```python
from build123d import *

# Parameters (mm, degrees)
TRIAL_LOAD_PLATE_PROFILE_R           = 13
TRIAL_LOAD_PLATE_PROFILE_R_2         = 4
TRIAL_LOAD_PLATE_DEPTH               = 4
CAPTURED_HORN_KEY_BOSS_START         = -1.65
CAPTURED_HORN_KEY_BOSS_PROFILE_R     = 13
CAPTURED_HORN_KEY_BOSS_DEPTH         = 1.65
KEY_POCKET_HUB_START                 = -1.65
STOCK_HORN_POCKET_HUB_R              = 3.5
KEY_POCKET_HUB_DEPTH                 = 1.65
KEY_POCKET_HORIZONTAL_START          = -1.65
STOCK_HORN_POCKET_HORIZONTAL_W       = 16.3
STOCK_HORN_POCKET_HORIZONTAL_H       = 4.1
KEY_POCKET_HORIZONTAL_DEPTH          = 1.65
KEY_POCKET_VERTICAL_START            = -1.65
STOCK_HORN_POCKET_VERTICAL_W         = 4.1
STOCK_HORN_POCKET_VERTICAL_H         = 16.3
KEY_POCKET_VERTICAL_DEPTH            = 1.65
KEY_POCKET_ROUNDED_TIPS_START        = -1.65
STOCK_HORN_POCKET_ROUNDED_TIPS_R     = 2.05
KEY_POCKET_ROUNDED_TIPS_DEPTH        = 1.65
UNMODIFIED_HORN_CAPTURE_M2_START     = -50
UNMODIFIED_HORN_CAPTURE_M2_PROFILE_R = 1.15
UNMODIFIED_HORN_CAPTURE_M2_DEPTH     = 69.814887722
HUB_CLEARANCE_IN_KEY_BOSS_ONLY_START = -1.65
HORN_CENTER_HUB_CLEARANCE_R          = 4
HUB_CLEARANCE_IN_KEY_BOSS_ONLY_DEPTH = 1.65


with BuildPart() as part:
    # Trial_load_plate_profile → Trial_load_plate (new body)
    with BuildSketch(Plane.XY):
        Circle(TRIAL_LOAD_PLATE_PROFILE_R)
        Circle(TRIAL_LOAD_PLATE_PROFILE_R_2, mode=Mode.SUBTRACT)
    extrude(amount=TRIAL_LOAD_PLATE_DEPTH)

    # Captured_horn_key_boss_profile → Captured_horn_key_boss (add)
    with BuildSketch(Plane.XY.offset(CAPTURED_HORN_KEY_BOSS_START)):
        Circle(CAPTURED_HORN_KEY_BOSS_PROFILE_R)
    extrude(amount=CAPTURED_HORN_KEY_BOSS_DEPTH)

    # Stock_horn_pocket_Hub → Key_pocket_Hub (cut)
    with BuildSketch(Plane.XY.offset(KEY_POCKET_HUB_START)):
        Circle(STOCK_HORN_POCKET_HUB_R)
    extrude(amount=KEY_POCKET_HUB_DEPTH, mode=Mode.SUBTRACT)

    # Stock_horn_pocket_Horizontal → Key_pocket_Horizontal (cut)
    with BuildSketch(Plane.XY.offset(KEY_POCKET_HORIZONTAL_START)):
        Rectangle(STOCK_HORN_POCKET_HORIZONTAL_W, STOCK_HORN_POCKET_HORIZONTAL_H)
    extrude(amount=KEY_POCKET_HORIZONTAL_DEPTH, mode=Mode.SUBTRACT)

    # Stock_horn_pocket_Vertical → Key_pocket_Vertical (cut)
    with BuildSketch(Plane.XY.offset(KEY_POCKET_VERTICAL_START)):
        Rectangle(STOCK_HORN_POCKET_VERTICAL_W, STOCK_HORN_POCKET_VERTICAL_H)
    extrude(amount=KEY_POCKET_VERTICAL_DEPTH, mode=Mode.SUBTRACT)

    # Stock_horn_pocket_Rounded_tips → Key_pocket_Rounded_tips (cut)
    with BuildSketch(Plane.XY.offset(KEY_POCKET_ROUNDED_TIPS_START)):
        with Locations((8.15, 0)):
            Circle(STOCK_HORN_POCKET_ROUNDED_TIPS_R)
        with Locations((-8.15, 0)):
            Circle(STOCK_HORN_POCKET_ROUNDED_TIPS_R)
        with Locations((0, 8.15)):
            Circle(STOCK_HORN_POCKET_ROUNDED_TIPS_R)
        with Locations((0, -8.15)):
            Circle(STOCK_HORN_POCKET_ROUNDED_TIPS_R)
    extrude(amount=KEY_POCKET_ROUNDED_TIPS_DEPTH, mode=Mode.SUBTRACT)

    # Unmodified_horn_capture_M2_profile → Unmodified_horn_capture_M2 (cut, through all)
    with BuildSketch(Plane.XY.offset(UNMODIFIED_HORN_CAPTURE_M2_START)):
        with Locations((7, 7)):
            Circle(UNMODIFIED_HORN_CAPTURE_M2_PROFILE_R)
        with Locations((-7, 7)):
            Circle(UNMODIFIED_HORN_CAPTURE_M2_PROFILE_R)
        with Locations((-7, -7)):
            Circle(UNMODIFIED_HORN_CAPTURE_M2_PROFILE_R)
        with Locations((7, -7)):
            Circle(UNMODIFIED_HORN_CAPTURE_M2_PROFILE_R)
    extrude(amount=UNMODIFIED_HORN_CAPTURE_M2_DEPTH, mode=Mode.SUBTRACT)

    # Horn_center_hub_clearance → Hub_clearance_in_key_boss_only (cut)
    with BuildSketch(Plane.XY.offset(HUB_CLEARANCE_IN_KEY_BOSS_ONLY_START)):
        with Locations(Location((0, 0, 0), (0, 0, 149.169502568))):
            Circle(HORN_CENTER_HUB_CLEARANCE_R)
    extrude(amount=HUB_CLEARANCE_IN_KEY_BOSS_ONLY_DEPTH, mode=Mode.SUBTRACT)


solid = part.part
```
Can you work these out from the model? Positions are in its coordinate system, mm. A direction names the side the tool comes from. Give positions to 0.01 mm unless a question says otherwise; leave off trailing zeros. Order: outer loops, then holes, each group sorted by start corner. A loop starts at its lowest first (then second) coordinate and runs counter-clockwise, first axis right, second up. Notation, with made-up numbers: (76, 46.5) - (116, 46.5) arc R28 cw to (116, 80.5) - close; hole circle Ø9 at (32, 83.5). An arc over 180 degrees is marked (long way). Use a Markdown table: item, result. Add a question column.
Q1. Please list where these lines run through material, in increasing order: line 1 along Y through (x, z) = (-7, 2.1); line 2 along X through (y, z) = (-3, 0.9).
Q2. I'm going to push flat-ended pins straight in: pin 1 (1.8 mm diameter, centred on x = -7, y = 7, fed in from -Z); pin 2 (0.5 mm diameter, centred on y = 6.5, z = -1, fed in from -X); pin 3 (2 mm diameter, centred on x = 1, y = -7, fed in from -Z); pin 4 (1.3 mm diameter, centred on x = -5, z = -0.5, fed in from -Y). Where does each tip first touch, or does it pass through?
Q3. If we section it at B-B on y = 2.75: Write out the boundary of the cut face in (x, z).
Q4. If we mould it in two halves opening along X, with no side actions, what happens to faces 1 (the cylindrical face through (10.2, 0, -0.8)), 2 (the flat face through (3, 3, 4)), 3 (the cylindrical face through (-10.316, -7.91, 1.135))? For each: released by +X, released by -X, zero draft, split by the parting line, or undercut.
Q5. If we section it at D-D on x = -7.5: Write out the boundary of the cut face in (y, z), plus the area to 3 significant figures.
Q6. If we section it at C-C on z = 2.2: Write out the boundary of the cut face in (x, y).
Q7. On a 3-axis mill with a long thin cutter (end or side, diameter ignored), from which of +Z, -Z, +X, -X, +Y, -Y can I reach the whole of each face in a straight line? I mean faces 4 (the cylindrical face through (6.85, -5.86, 1.14)), 5 (the flat face through (-2.05, -6, -1)). Say none if no direction works.
Q8. If we section it at A-A on x = 0: Write out the boundary of the cut face in (y, z).
Answers follow:
| question | item | result |
|---|---|---|
| 1 | line 1 | y = -10.95 to -8.15, -5.85 to 5.85, 8.15 to 10.95 |
| 1 | line 2 | x = -12.65 to -2.65, 2.65 to 12.65 |
| 2 | pin 1 | passes through |
| 2 | pin 2 | stops at x = -11.4 |
| 2 | pin 3 | stops at z = 0 |
| 2 | pin 4 | stops at y = -12.25 |
| 3 | outline | (-12.71, -1.65) - (-2.9, -1.65) - (-2.9, 4) - (-12.71, 4) - close; (2.9, -1.65) - (12.71, -1.65) - (12.71, 4) - (2.9, 4) - close |
| 4 | face 1 | undercut |
| 4 | face 2 | zero draft |
| 4 | face 3 | split by the parting line |
| 5 | outline | (-10.62, -1.65) - (-8.04, -1.65) - (-8.04, 4) - (-10.62, 4) - close; (-5.96, -1.65) - (-2.05, -1.65) - (-2.05, 0) - (2.05, 0) - (2.05, -1.65) - (5.96, -1.65) - (5.96, 4) - (-5.96, 4) - close; (8.04, -1.65) - (10.62, -1.65) - (10.62, 4) - (8.04, 4) - close |
| 5 | area | 89.8 mm^2 |
| 6 | outline | circle Ø26 at (0, 0); hole circle Ø2.3 at (-7, -7); hole circle Ø2.3 at (-7, 7); hole circle Ø8 at (0, 0); hole circle Ø2.3 at (7, -7); hole circle Ø2.3 at (7, 7) |
| 7 | face 4 | +Z, -Z |
| 7 | face 5 | -Z |
| 8 | outline | (-13, -1.65) - (-10.2, -1.65) - (-10.2, 0) - (-4, 0) - (-4, 4) - (-13, 4) - close; (4, 0) - (10.2, 0) - (10.2, -1.65) - (13, -1.65) - (13, 4) - (4, 4) - close |
